Geometry: final body of the model. Coordinates: model frame, mm. A direction names the side the tool comes from. Give positions to 0.01 mm unless a question says otherwise; leave off trailing zeros. Loops run counter-clockwise (first coordinate to the right, second up) from the corner with the lowest first, then second, coordinate; pieces in that order, holes last. Notation, with made-up numbers: M 77.5,-12.5 L 123.5,-12.5 A17 ccw 123.5,16.5 Z; hole C 31.5,64 d5. An arc over 180 degrees is marked long. Put each result on its own line as item: value.
```python
from build123d import *

# Parameters (mm, degrees)
F1_DEPTH = 50.8
F2_T     = -2.54


with BuildPart() as f1:
    # F0 (on Front) → F1 (new body)
    with BuildSketch(Plane.XZ):
        Polygon((-30.403135, 62.145095), (-145.066381, 62.145095), (-145.066381, -55.625658), (-109.885611, -55.625658), (-109.885611, -13.436122), (-63.846581, -13.436122), (-63.846581, -55.625658), (-30.403135, -55.625658), align=None)
    extrude(amount=F1_DEPTH)

    # F2
    f2_openings = [f1.faces().sort_by_distance(p)[0] for p in [
        (-86.866096, -25.4, -13.436122),
        (-109.885611, -25.4, -34.53089),
        (-63.846581, -25.4, -34.53089),
        (-127.475996, -25.4, -55.625658),
        (-47.124858, -25.4, -55.625658),
    ]]
    offset(amount=F2_T, openings=f2_openings)


solid = f1.part
```
Item 1: Mould query, pull axis X, two halves, no side actions, for faces 1 (the flat face through (-142.526, -25, 3)), 2 (the flat face through (-145.066, -25, 4)), 3 (the flat face through (-143, -25, -55.626)). Classes: pulls with the +X half, pulls with the -X half, needs draft (parallel to the pull), parting line crosses it, or undercut.
Output values:
face 1: undercut
face 2: pulls with the -X half
face 3: needs draft
Item 2: Line query: probe 1 along X at (y, z) = (-32.5, -11); probe 2 along Y at (x, z) = (-49, 46.5); probe 3 along Z at (x, y) = (-81, -32.5). Output: solid intervals per line, ascending. Write a range as [from, to].
Output values:
probe 1: [-145.07, -142.53], [-32.94, -30.4]
probe 2: [-50.8, -48.26], [-2.54, 0]
probe 3: [59.61, 62.15]
Item 3: Set-up query: faces 4 (the flat face through (-30.403, -25, 2)), 5 (the flat face through (-32.943, -25, 1)). Return all of +Z, -Z, +X, -X, +Y, -Y with unobstructed straight access to the full face (end or side cutting, diameter ignored); none if empty.
Output values:
face 4: +Z, -Z, +X, +Y, -Y
face 5: -Z
Item 4: Section D-D on y = -29.5. Output: boundary loops of the cut face in (x, z), then the cut area to 3 significant figures.
Output values:
outline: M -145.07,-55.63 L -142.53,-55.63 L -142.53,59.61 L -32.94,59.61 L -32.94,-55.63 L -30.4,-55.63 L -30.4,62.15 L -145.07,62.15 Z
area: 877 mm²
Item 5: Section C-C on z = 20. Output: boundary loops of the cut face in (x, y).
Output values:
outline: M -145.07,-50.8 L -30.4,-50.8 L -30.4,0 L -145.07,0 Z; hole M -142.53,-48.26 L -32.94,-48.26 L -32.94,-2.54 L -142.53,-2.54 Z
Item 6: Pin query (flat end, axial travel): pin 1 Ø5 at (x, y) = (-67, -34) entering from -Z; pin 2 Ø3 at (x, y) = (-86.5, -49.5) entering from -Z. Return the tip coordinate at first contact, or that it passes through.
Output values:
pin 1: z = 59.61
pin 2: z = -13.44
Item 7: Section A-A on z = -35.5. Output: boundary loops of the cut face in (x, y), then the cut area to 3 significant figures.
Output values:
outline: M -145.07,-50.8 L -109.89,-50.8 L -109.89,-48.26 L -142.53,-48.26 L -142.53,-2.54 L -109.89,-2.54 L -109.89,0 L -145.07,0 Z; M -63.85,-50.8 L -30.4,-50.8 L -30.4,0 L -63.85,0 L -63.85,-2.54 L -32.94,-2.54 L -32.94,-48.26 L -63.85,-48.26 Z
area: 581 mm²
Item 8: Section B-B on x = -42.5. Output: boundary loops of the cut face in (y, z).
Output values:
outline: M -50.8,-55.63 L -48.26,-55.63 L -48.26,59.61 L -2.54,59.61 L -2.54,-55.63 L 0,-55.63 L 0,62.15 L -50.8,62.15 Z
